from build123d import *

# Parameters (mm, degrees)
SKETCH1_R           = 3.175
SKETCH1_R_2         = 1.5875
BOSS_EXTRUDE1_DEPTH = 2.4765


with BuildPart() as part:
    # Sketch1 → Boss-Extrude1 (new, symmetric)
    with BuildSketch(Plane(origin=(0, 0, 0), x_dir=(1, 0, 0), z_dir=(0, 1, 0))):
        with BuildLine():
            Line((34.700549349, -12.916534941), (61.399556839, -22.854667611))
            ThreePointArc((61.399556839, -22.854667611), (55.420174256, -34.940602415), (47.093148029, -45.546424892))
            ThreePointArc((47.093148029, -45.546424892), (15.086508303, -14.560725649), (-28.536322062, -23.593289791))
            Line((-28.536322062, -23.593289791), (-50.492501165, -41.746242199))
            ThreePointArc((-50.492501165, -41.746242199), (-57.969536443, -30.52497758), (-62.990935022, -18.010650091))
            ThreePointArc((-62.990935022, -18.010650091), (-20.153212462, -5.78493662), (-6.164227287, 36.509824732))
            Line((-6.164227287, 36.509824732), (-10.907055674, 64.600909809))
            ThreePointArc((-10.907055674, 64.600909809), (2.549362187, 65.465579995), (15.897786993, 63.557074983))
            ThreePointArc((15.897786993, 63.557074983), (5.066704158, 20.34566227), (34.700549349, -12.916534941))
        make_face()
        Circle(SKETCH1_R, mode=Mode.SUBTRACT)
        with Locations((-1.743506635, 58.073174541)):
            Circle(SKETCH1_R_2, mode=Mode.SUBTRACT)
        with Locations((-49.421091113, -30.546508308)):
            Circle(SKETCH1_R_2, mode=Mode.SUBTRACT)
        with Locations((51.164597749, -27.526666233)):
            Circle(SKETCH1_R_2, mode=Mode.SUBTRACT)
    extrude(amount=BOSS_EXTRUDE1_DEPTH, both=True)


solid = part.part
Could you check a few things on this model? Use its own coordinates, in mm. A direction names the side the tool comes from. Give positions to 0.01 mm unless a question says otherwise; leave off trailing zeros. Order: outer loops, then holes, each group sorted by start corner. A loop starts at its lowest first (then second) coordinate and runs counter-clockwise, first axis right, second up.
1. For faces 1 (the cylindrical face through (-20.625, 0.035, 6.231)), 2 (the flat face through (-8.502, 0.035, -50.359)), which set-ups out of +Z, -Z, +X, -X, +Y, -Y let a thin tool reach every point of the face, with its end or its side?
2. Suppose I cut it at C-C (y = 0.95). Give the number of separate pieces and of enclosed holes in the cut face, plus the area to 3 significant figures.
3. Suppose I cut it at A-A (z = 0). List the corners of the cut face in (x, y) for me (1 decimal).
4. Will these pins go through, and if not, where does the flat tip stop? P1, Ø1.9, axis at x = 51.16, z = 27.53, coming from the -Y side; P2, Ø1, axis at x = 30, y = 0, coming from the +Z side; P3, Ø2, axis at x = -49.5, y = 1, coming from the -Z side; P4, Ø2, axis at x = -21.5, y = 1.5, coming from the +Z side.
5. Suppose I cut it at B-B (x = 14). List the corners of the cut face in (y, z) for me.
6. I need wall thicknesses on L1, parallel to X at y = -0.2, z = 31.5; L2, parallel to Z at x = 14, y = -1.45; L3, parallel to X at y = -1.3, z = -58. Which ranges of each line are inside material? Lowest first, please.
7. We'd pull the mould along X, two halves only. Please class faces 3 (the flat face through (-39.36, 0.03, 32.54)), 4 (the cylindrical face through (2.36, 0.035, -65.473)), 5 (the cylindrical face through (49.905, -0.035, 28.493)), 6 (the cylindrical face through (4.916, 0.035, -20.977)): pulls with the +X half, pulls with the -X half, needs draft (parallel to the pull), parting line crosses it, or undercut.
8. Suppose I cut it at D-D (z = -17.5). List the corners of the cut face in (x, y) for me.
Solved:
1. face 1: +Y, -Y
1. face 2: -X, +Y, -Y
2. separate pieces: 1
2. enclosed holes: 4
2. area: 2,760 mm2
3. outline: (-15, -2.5) - (-3.2, -2.5) - (-3.2, 2.5) - (-15, 2.5) - close; (3.2, -2.5) - (15.8, -2.5) - (15.8, 2.5) - (3.2, 2.5) - close
4. P1: passes through
4. P2: stops at z = 22.28
4. P3: stops at z = 18.82
4. P4: stops at z = 19.34
5. outline: (-2.48, -64) - (2.48, -64) - (2.48, -61.31) - (-2.48, -61.31) - close; (-2.48, -2.12) - (2.48, -2.12) - (2.48, 14.26) - (-2.48, 14.26) - close
6. L1: x = -57.45 to -50.69, -48.15 to -38.1, 39.74 to 57.45
6. L2: z = -64 to -61.31, -2.12 to 14.26
6. L3: x = -9.79 to -3.33, -0.16 to 11.6
7. face 3: undercut
7. face 4: parting line crosses it
7. face 5: undercut
7. face 6: pulls with the +X half
8. outline: (-6.81, -2.48) - (5.86, -2.48) - (5.86, 2.48) - (-6.81, 2.48) - close
